Geometry: see drawing. Coordinates: mm, zero at the bounding-box minimum. A direction names the side the tool comes from. Give positions to 0.01 mm unless a question says otherwise; leave off trailing zeros. Order: outer loops, then holes, each group sorted by start corner. A loop starts at its lowest first (then second) coordinate and runs counter-clockwise, first axis right, second up. Notation, with made-up numbers: M 89.5,61.5 L 97.5,61.5 A11 cw 97.5,70.5 Z; hole C 79,40.5 d7. An arc over 180 degrees is marked long. Return JSON: item names as keys, results as strings.
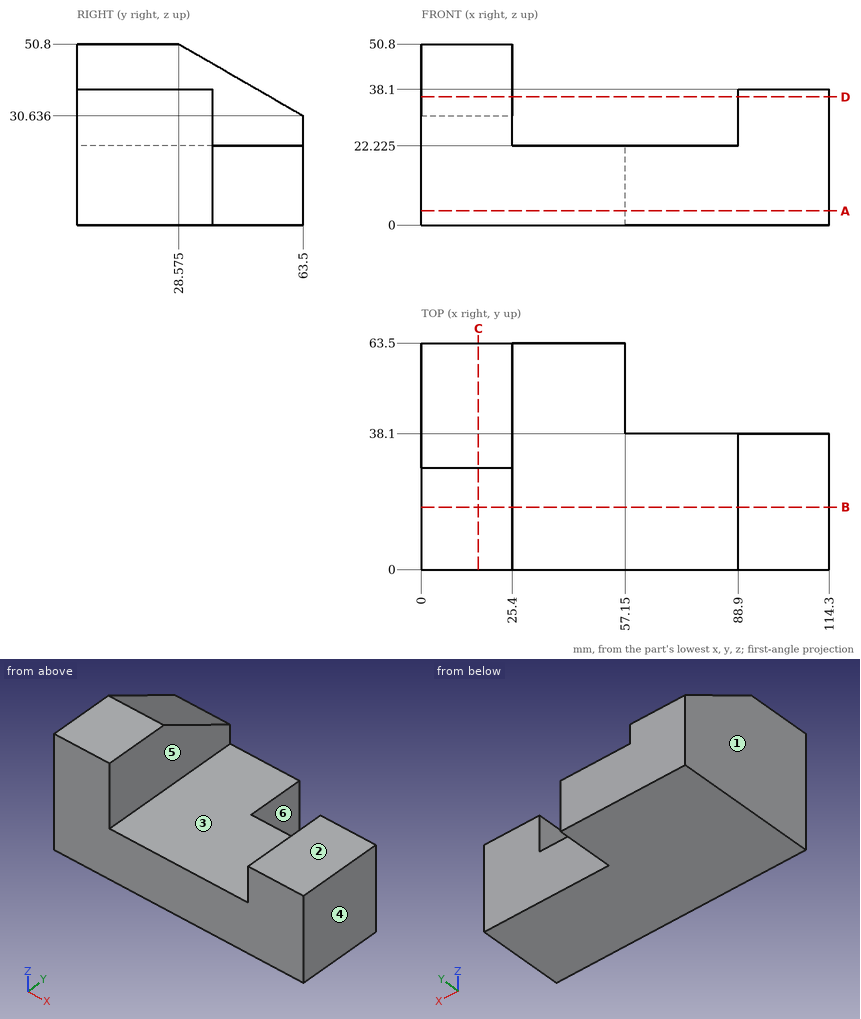
1. Section query D-D (z = 36). Return loops of the section in (x, y), then the cut area to 3 significant figures.
Evaluation:
{"outline": "M 0,0 L 25.4,0 L 25.4,54.21 L 0,54.21 Z; M 88.9,0 L 114.3,0 L 114.3,38.1 L 88.9,38.1 Z", "area": "2,340 mm^2"}
2. Set-up query: the marked faces 4, 5 and 6. Return all of +Z, -Z, +X, -X, +Y, -Y with unobstructed straight access to the full face (end or side cutting, diameter ignored); none if empty.
Evaluation:
{"face 4": "+Z, -Z, +X, +Y, -Y", "face 5": "+Z, +Y, -Y", "face 6": "+Z, -Z, +X, +Y"}
3. Section query B-B (y = 17.5). Return loops of the section in (x, z) (3 decimals), then the cut area to 3 significant figures.
Evaluation:
{"outline": "M 0,0 L 114.3,0 L 114.3,38.1 L 88.9,38.1 L 88.9,22.225 L 25.4,22.225 L 25.4,50.8 L 0,50.8 Z", "area": "3,670 mm^2"}
4. Section query A-A (z = 4). Return loops of the section in (x, y), then the cut area to 3 significant figures.
Evaluation:
{"outline": "M 0,0 L 114.3,0 L 114.3,38.1 L 57.15,38.1 L 57.15,63.5 L 0,63.5 Z", "area": "5,810 mm^2"}
5. Section query C-C (x = 16). Return loops of the section in (y, z) (3 decimals).
Evaluation:
{"outline": "M 0,0 L 63.5,0 L 63.5,30.636 L 28.575,50.8 L 0,50.8 Z"}
6. First-contact query: pin 1 (18 mm diameter, centred on y = 55, z = 9, fed in from +X); pin 2 (12 mm diameter, centred on x = 63.5, z = 9, fed in from +Y); pin 3 (10 mm diameter, centred on x = 36.5, y = 44, fed in from +Z) (3 decimals); pin 4 (8 mm diameter, centred on x = 13, z = 34, fed in from -Y). Flat tips, straight axial feed; report the tip coordinate or a pass-through.
Evaluation:
{"pin 1": "stops at x = 57.15", "pin 2": "stops at y = 38.1", "pin 3": "stops at z = 22.225", "pin 4": "stops at y = 0"}
7. Draft query along X for the marked faces 1, 2 and 3. Return one class per face: pulls with the +X half, pulls with the -X half, needs draft (parallel to the pull), parting line crosses it, or undercut.
Evaluation:
{"face 1": "pulls with the -X half", "face 2": "needs draft", "face 3": "undercut"}
8. Ray query, probe 1 along X at (y, z) = (6, 23); probe 2 along X at (y, z) = (50, 11.5); probe 3 along X at (y, z) = (3, 48). Return the intervals inside material, ascending.
Evaluation:
{"probe 1": "x = 0 to 25.4, 88.9 to 114.3", "probe 2": "x = 0 to 57.15", "probe 3": "x = 0 to 25.4"}
